Could you check a few things on this model? Use its own coordinates, in mm. Face numbers are marked on the shaded views. A direction names the side the tool comes from. Coordinates: 2 decimals unless noted, no trailing zeros. Order: outer loops, then holes, each group sorted by start corner. A loop starts at its lowest first (then second) coordinate and runs counter-clockwise, first axis right, second up. Notation, with made-up numbers: (35.5, 73.25) - (43.5, 73.25) arc R14 ccw to (43.5, 86.25) - close; hole circle Ø5 at (-14.5, 29.25). An arc over 180 degrees is marked (long way). Answer as CSV lines item,"result". Start each with the question number.
1. Thinking about a two-plate mould opening in Z: for the marked faces 3, 4 and 5, which applies, released by +Z, released by -Z, zero draft, split by the parting line, or undercut?
2. I want a section at B-B, the plane z = 6. List the corners of the cut face in (x, y) for me, and give its area (3 significant figures).
3. For pin 1 (1.5 mm diameter, centred on x = -5.5, z = 6.5, fed in from -Y); pin 2 (4 mm diameter, centred on y = 0.5, z = 7, fed in from -X), each with a flat end and sliding along its axis, tell me the tip position at first contact or that it passes through.
4. I want a section at D-D, the plane x = -4.5. List the corners of the cut face in (y, z) for me, and give its area (3 significant figures).
5. For the marked faces 1 and 2, which set-ups out of +Z, -Z, +X, -X, +Y, -Y let a thin tool reach every point of the face, with its end or its side?
6. I need wall thicknesses on probe 1 along Y at (x, z) = (0.85, 6); probe 2 along Y at (x, z) = (0, 1); probe 3 along Y at (x, z) = (1.2, 6). Which ranges of each line are inside material? Lowest first, please.
7. I want a section at A-A, the plane x = 0. List the corners of the cut face in (y, z) for me.
8. I want a section at C-C, the plane y = 0. List the corners of the cut face in (x, z) for me.
from build123d import *

# Parameters (mm, degrees)
SKETCH1_R           = 2.15
BOSS_EXTRUDE1_DEPTH = 12
SKETCH2_W           = 7.5
SKETCH2_H           = 7.5
SKETCH2_R           = 2.5
CUT_EXTRUDE1_DEPTH  = 5
SKETCH2_2_R         = 2.5
CUT_EXTRUDE2_DEPTH  = 13
SKETCH3_R           = 4.05
CUT_EXTRUDE3_DEPTH  = 3


with BuildPart() as part:
    # Sketch1 → Boss-Extrude1 (new body)
    with BuildSketch(Plane.XY):
        with BuildLine():
            Line((-4, -10), (2, -10))
            ThreePointArc((2, -10), (4.121320344, -9.121320344), (5, -7))
            Line((5, -7), (5, 7))
            ThreePointArc((5, 7), (4.121320344, 9.121320344), (2, 10))
            Line((2, 10), (-4, 10))
            ThreePointArc((-4, 10), (-6.121320344, 9.121320344), (-7, 7))
            Line((-7, 7), (-7, -7))
            ThreePointArc((-7, -7), (-6.121320344, -9.121320344), (-4, -10))
        make_face()
        with Locations((0, 5)):
            Circle(SKETCH1_R, mode=Mode.SUBTRACT)
        with Locations((0, -5)):
            Circle(SKETCH1_R, mode=Mode.SUBTRACT)
    extrude(amount=BOSS_EXTRUDE1_DEPTH)

    # Sketch2 → Cut-Extrude1 (cut)
    with BuildSketch(Plane.ZY.offset(7)):
        with Locations((6, 0)):
            Rectangle(SKETCH2_W, SKETCH2_H)
        with Locations((6, 0)):
            Circle(SKETCH2_R, mode=Mode.SUBTRACT)
    extrude(amount=-CUT_EXTRUDE1_DEPTH, mode=Mode.SUBTRACT)

    # Sketch2<2> → Cut-Extrude2 (cut, through all)
    with BuildSketch(Plane.ZY.offset(7)):
        with Locations((6, 0)):
            Circle(SKETCH2_2_R)
    extrude(amount=-CUT_EXTRUDE2_DEPTH, mode=Mode.SUBTRACT)

    # Sketch3 → Cut-Extrude3 (cut)
    with BuildSketch(Plane(origin=(5, 0, 0), x_dir=(0, 0, -1), z_dir=(1, 0, 0))):
        with Locations((-6, 0)):
            Circle(SKETCH3_R)
    extrude(amount=-CUT_EXTRUDE3_DEPTH, mode=Mode.SUBTRACT)


solid = part.part
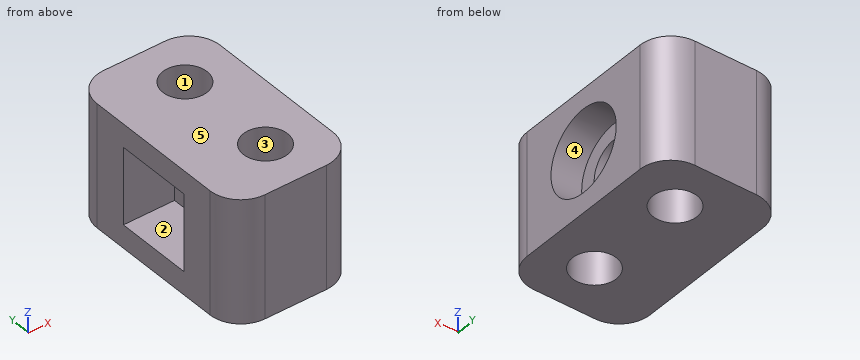
Solved:
1,face 3,"zero draft"
1,face 4,"undercut"
1,face 5,"released by +Z"
2,outline,"(-7, -7) arc R3 ccw to (-4, -10) - (2, -10) arc R3 ccw to (5, -7) - (5, -4.05) - (2, -4.05) - (2, -2.5) - (-2, -2.5) - (-2, -3.75) - (-7, -3.75) - close; (-7, 3.75) - (-2, 3.75) - (-2, 2.5) - (2, 2.5) - (2, 4.05) - (5, 4.05) - (5, 7) arc R3 ccw to (2, 10) - (-4, 10) arc R3 ccw to (-7, 7) - close; hole circle Ø4.3 at (0, -5); hole circle Ø4.3 at (0, 5)"
2,area,"121 mm2"
3,pin 1,"stops at y = -9.9"
3,pin 2,"stops at x = -2"
4,outline,"(-9.96, 0) - (9.96, 0) - (9.96, 12) - (-9.96, 12) - close; hole (-3.75, 2.25) - (3.75, 2.25) - (3.75, 9.75) - (-3.75, 9.75) - close"
4,area,"183 mm2"
5,face 1,"+Z, -Z"
5,face 2,"-X"
6,probe 1,"y = -10 to -6.97, -3.03 to -2.5, 2.5 to 3.03, 6.97 to 10"
6,probe 2,"y = -10 to -7.15, -2.85 to 2.85, 7.15 to 10"
6,probe 3,"y = -10 to -6.78, -3.22 to -2.5, 2.5 to 3.22, 6.78 to 10"
7,outline,"(-10, 0) - (-7.15, 0) - (-7.15, 12) - (-10, 12) - close; (-2.85, 0) - (2.85, 0) - (2.85, 12) - (-2.85, 12) - close; (7.15, 0) - (10, 0) - (10, 12) - (7.15, 12) - close; hole circle Ø5 at (0, 6)"
8,outline,"(-7, 0) - (5, 0) - (5, 1.95) - (2, 1.95) - (2, 3.5) - (-2, 3.5) - (-2, 2.25) - (-7, 2.25) - close; (-7, 9.75) - (-2, 9.75) - (-2, 8.5) - (2, 8.5) - (2, 10.05) - (5, 10.05) - (5, 12) - (-7, 12) - close"
